Autodesk Inventor part; units mm, degrees
ref_plane "Cross Section Plane" through (-117.4632, -128.8972, 0) normal (0.7071, 0.7071, 0) x (0, 0, 1)
ref_plane "Work Plane2" through (-123.1802, -123.1802, 0) normal (-1, 0, 0) x (0, 0, 1)
ref_plane "Work Plane3" through (-80.7538, -80.7538, 0) normal (-0.8049, -0.5934, 0) x (0, 0, 1)
sketch "Sketch Path" plane through (0, 0, 0) normal (0, 0, 1) x (1, 0, 0)
  arc A0 (-128.8972, -117.4632) -> (-117.4632, -128.8972) centre (-123.1802, -123.1802) ccw
  arc A1 (-75.0368, -86.4708) -> (-86.4708, -75.0368) centre (-80.7538, -80.7538) ccw
  line L0 (-75.0368, -86.4708) -> (-117.4632, -128.8972)
  line L1 (-128.8972, -117.4632) -> (-86.4708, -75.0368)
ref_plane "Cross Section Plane" through (-117.4632, -128.8972, 0) normal (0.7071, 0.7071, 0) x (0, 0, 1)
ref_plane "Work Plane2" through (-123.1802, -123.1802, 0) normal (-1, 0, 0) x (0, 0, 1)
ref_plane "Work Plane3" through (-80.7538, -80.7538, 0) normal (-0.8049, -0.5934, 0) x (0, 0, 1)
sketch "Cross Section" plane through (-117.4632, -128.8972, 0) normal (0.7071, 0.7071, 0) x (0, 0, 1)
  line L0 (-3.175, 0.381) -> (3.175, 0.381)
  line L1 (3.175, 0.381) -> (3.175, -0.254)
  line L2 (3.175, -0.254) -> (-3.175, -0.254)
  line L3 (-3.175, -0.254) -> (-3.175, 0.381)
  line L4 (-3.175, 0) -> (3.175, 0) construction
  point P0 (0, 0)
  point P1 (0, 0)
  dimension "d0" = 6.35
  dimension "d4" = 0.254
  dimension "d5" = 0.381
sweep "Belt" add profiles "Cross Section" path "Sketch Path"
equation "\"d0\" = da_B"
equation "\"d4\" = da_a"
equation "\"d5\" = da_a2"
equation "\"da_B\" = 6.35"
equation "\"da_pb\" = 2.032"
equation "\"da_L\" = 170.8"
equation "\"da_a\" = 0.254"
equation "\"da_S\" = 1.143"
equation "\"da_Beta\" = 20deg"
equation "\"da_Ht\" = 0.508"
equation "\"da_H\" = 1.143"
equation "\"da_a2\" = 0.381"
properties part number "Synchronous Belt" material "Rubber"
Build history of the part. All positions in model axes, mm. A direction names the side the tool comes from. Coordinates: 2 decimals unless noted, no trailing zeros. Order: outer loops, then holes, each group sorted by start corner. A loop starts at its lowest first (then second) coordinate and runs counter-clockwise, first axis right, second up. Notation, with made-up numbers: (-18.5, 15) - (3.5, 15) arc R33 ccw to (3.5, 46) - close; hole circle Ø2 at (24.5, 75). An arc over 180 degrees is marked (long way). Put each result on its own line as item: value.
1. Drop flat-ended pins along their axis: P1, Ø5, axis at x = -88.5, y = -103.5, coming from the -Z side (3 decimals); P2, Ø3, axis at y = -116, z = 2.5, coming from the +X side. Give the stop position or say it passes through.
Answer sheet:
P1: stops at z = -3.175
P2: stops at x = -102.53
2. Saw through at C-C (y = -80). Write the cut outline in (x, z) (3 decimals), and give its area (3 significant figures).
Answer sheet:
outline: (-91.973, -3.175) - (-91.075, -3.175) - (-91.075, 3.175) - (-91.973, 3.175) - close; (-72.959, -3.175) - (-72.321, -3.175) - (-72.321, 3.175) - (-72.959, 3.175) - close
area: 9.75 mm^2
3. Probe line 1 along X through (y, z) = (-84, 0.5); line 2 along Y through (x, z) = (-122.5, -2.5); line 3 along X through (y, z) = (-123, 1). List the from-to ranges inside material, lowest first. Write a range as [from, to].
Answer sheet:
line 1: x = [-95.97, -95.07], [-73.63, -72.93]
line 2: y = [-131.62, -130.98], [-111.43, -110.53]
line 3: x = [-131.64, -131.01], [-111.93, -111.03]
4. Tool access for faces 1 (the face through (-107.6, -96.1, 3.175)), 2 (the face through (-107.801, -96.727, -0.044)): list every direction of +Z, -Z, +X, -X, +Y, -Y with a clear straight run to the whole face (end or side of a thin tool).
Answer sheet:
face 1: +Z, +X, -X, +Y, -Y
face 2: +Z, -Z
5. Saw through at A-A (z = 1.75). Write the cut outline in (x, y), and give its area (3 significant figures).
Answer sheet:
outline: (-129.17, -117.19) arc R8.47 ccw to (-117.19, -129.17) - (-74.77, -86.74) arc R8.47 ccw to (-86.74, -74.77) - close; hole (-128.72, -117.64) arc R7.83 ccw to (-117.64, -128.72) - (-75.22, -86.29) arc R7.83 ccw to (-86.29, -75.22) - close
area: 109 mm^2
6. Saw through at B-B (x = -76.5). Write the cut outline in (y, z) (3 decimals), and give its area (3 significant figures).
Answer sheet:
outline: (-88.473, -3.175) - (-87.575, -3.175) - (-87.575, 3.175) - (-88.473, 3.175) - close; (-74.179, -3.175) - (-73.434, -3.175) - (-73.434, 3.175) - (-74.179, 3.175) - close
area: 10.4 mm^2
7. Pull direction Y, two halves, no side cores. Call faces 3 (the face through (-95.684, -107.656, 0.044)), 4 (the face through (-74.9, -74.64, -0.04)), 5 (the face through (-75.096, -75.34, 0.044)): pulls with the +Y half, pulls with the -Y half, needs draft (parallel to the pull), parting line crosses it, or undercut.
Answer sheet:
face 3: pulls with the -Y half
face 4: parting line crosses it
face 5: undercut
